from build123d import *

# Parameters (mm, degrees)
BOSS_EXTRUDE1_DEPTH       = 280
SKETCH4_R                 = 15
BOSS_EXTRUDE2_DEPTH       = 15
CUT_EXTRUDE1_DEPTH        = 15
CUT_EXTRUDE2_DEPTH        = 15
SKETCH9_R                 = 15
CUT_EXTRUDE3_DEPTH        = 15
LPATTERN1_COUNT           = 2
LPATTERN1_PITCH           = 180
LPATTERN2_COUNT           = 2
LPATTERN2_PITCH           = 220
LPATTERN2_COPY_1_SKETCH_R = 15
LPATTERN2_COPY_1_DEPTH    = 15


with BuildPart() as part:
    # Sketch1 → Boss-Extrude1 (new body)
    with BuildSketch(Plane.XY):
        with BuildLine():
            Line((-120, 0), (120, 0))
            Line((120, 0), (120, 15))
            Line((120, 15), (37.749172176, 15))
            ThreePointArc((37.749172176, 15), (54.444104817, 62.799964787), (25, 103.989794856))
            Line((25, 103.989794856), (10, 103.989794856))
            Line((10, 103.989794856), (10, 93.729833462))
            ThreePointArc((10, 93.729833462), (0, 15), (-10, 93.729833462))
            Line((-10, 93.729833462), (-10, 103.989794856))
            Line((-10, 103.989794856), (-25, 103.989794856))
            ThreePointArc((-25, 103.989794856), (-54.444104817, 62.799964787), (-37.749172176, 15))
            Line((-37.749172176, 15), (-120, 15))
            Line((-120, 15), (-120, 0))
        make_face()
    extrude(amount=BOSS_EXTRUDE1_DEPTH)

    # Sketch4 → Boss-Extrude2 (add)
    with BuildSketch(Plane(origin=(-10, 0, 0), x_dir=(0, 0, -1), z_dir=(1, 0, 0))):
        with BuildLine():
            Line((-258.604852185, 154.832655732), (-258.604852185, 103.989794856))
            Line((-258.604852185, 103.989794856), (-198.604852185, 103.989794856))
            Line((-198.604852185, 103.989794856), (-198.604852185, 154.832655732))
            ThreePointArc((-198.604852185, 154.832655732), (-228.604852185, 184.832655732), (-258.604852185, 154.832655732))
        make_face()
        with Locations((-228.604852185, 154.832655732)):
            Circle(SKETCH4_R, mode=Mode.SUBTRACT)
        with BuildLine():
            Line((-81.395147815, 103.989794856), (-21.395147815, 103.989794856))
            Line((-21.395147815, 103.989794856), (-21.395147815, 154.832655732))
            ThreePointArc((-21.395147815, 154.832655732), (-51.395147815, 184.832655732), (-81.395147815, 154.832655732))
            Line((-81.395147815, 154.832655732), (-81.395147815, 103.989794856))
        make_face()
        with Locations((-51.395147815, 154.832655732)):
            Circle(SKETCH4_R, mode=Mode.SUBTRACT)
    boss_extrude2 = extrude(amount=-BOSS_EXTRUDE2_DEPTH)

    # Mirror1: Boss-Extrude2 across plane
    add(boss_extrude2.mirror(Plane(origin=(0, 0, 0), x_dir=(0, 0, 1), z_dir=(1, 0, 0))))

    # Sketch5 → Cut-Extrude1 (cut)
    with BuildSketch(Plane(origin=(0, 15, 0), x_dir=(1, 0, 0), z_dir=(0, 1, 0))):
        with BuildLine():
            Line((120, -250), (120, -30.000000185))
            ThreePointArc((120, -30.000000185), (111.21320337, -51.213203501), (90, -60))
            Line((90, -60), (37.749172176, -60))
            Line((37.749172176, -60), (37.749172176, -220))
            Line((37.749172176, -220), (90, -220))
            ThreePointArc((90, -220), (111.213203436, -228.786796564), (120, -250))
        make_face()
        with BuildLine():
            Line((120, 0), (90, 0))
            ThreePointArc((90, 0), (111.213203501, -8.78679663), (120, -30.000000185))
            Line((120, -30.000000185), (120, 0))
        make_face()
        with BuildLine():
            Line((120, -280), (120, -250))
            ThreePointArc((120, -250), (111.213203436, -271.213203436), (90, -280))
            Line((90, -280), (120, -280))
        make_face()
    extrude(amount=-CUT_EXTRUDE1_DEPTH, mode=Mode.SUBTRACT)

    # Sketch7 → Cut-Extrude2 (cut)
    with BuildSketch(Plane(origin=(0, 15, 0), x_dir=(1, 0, 0), z_dir=(0, 1, 0))):
        with BuildLine():
            Line((-37.749172176, -220), (-37.749172176, -60))
            Line((-37.749172176, -60), (-90, -60))
            ThreePointArc((-90, -60), (-111.213203468, -51.213203403), (-120, -29.999999908))
            Line((-120, -29.999999908), (-120, -250))
            ThreePointArc((-120, -250), (-111.213203436, -228.786796564), (-90, -220))
            Line((-90, -220), (-37.749172176, -220))
        make_face()
        with BuildLine():
            ThreePointArc((-120, -29.999999908), (-111.213203403, -8.786796532), (-90, 0))
            Line((-90, 0), (-120, 0))
            Line((-120, 0), (-120, -29.999999908))
        make_face()
        with BuildLine():
            ThreePointArc((-90, -280), (-111.213203436, -271.213203436), (-120, -250))
            Line((-120, -250), (-120, -280))
            Line((-120, -280), (-90, -280))
        make_face()
    extrude(amount=-CUT_EXTRUDE2_DEPTH, mode=Mode.SUBTRACT)

    # Sketch9 → Cut-Extrude3 (cut)
    with BuildSketch(Plane(origin=(0, 15, 0), x_dir=(1, 0, 0), z_dir=(0, 1, 0))):
        with Locations((90, -30)):
            Circle(SKETCH9_R)
    cut_extrude3 = extrude(amount=-CUT_EXTRUDE3_DEPTH, mode=Mode.SUBTRACT)

    # LPattern1: Cut-Extrude3 ×2
    with Locations(*[(-i * LPATTERN1_PITCH, 0, 0) for i in range(1, LPATTERN1_COUNT)]):
        add(cut_extrude3, mode=Mode.SUBTRACT)

    # LPattern2: Cut-Extrude3 ×2
    with Locations(*[(0, 0, i * LPATTERN2_PITCH) for i in range(1, LPATTERN2_COUNT)]):
        add(cut_extrude3, mode=Mode.SUBTRACT)

    # LPattern2 copy 1 sketch → LPattern2 copy 1 (cut)
    with BuildSketch(Plane(origin=(-180, 15, 220), x_dir=(1, 0, 0), z_dir=(0, 1, 0))):
        with Locations((90, -30)):
            Circle(LPATTERN2_COPY_1_SKETCH_R)
    extrude(amount=-LPATTERN2_COPY_1_DEPTH, mode=Mode.SUBTRACT)


solid = part.part
Geometry: final body of the model. Coordinates: model frame, mm. A direction names the side the tool comes from. Round coordinates to 2 decimals unless told otherwise and drop trailing zeros. Loops run counter-clockwise (first coordinate to the right, second up) from the corner with the lowest first, then second, coordinate; pieces in that order, holes last. Notation, with made-up numbers: M 70.25,67 L 93.25,67 A24 ccw 93.25,98 Z; hole C -21.75,-34 d6. An arc over 180 degrees is marked long. One line per question, with ' | ' between items.
(1) Cut plane A-A on y = 55. Return the cut outline in (x, z).
Check result:
outline: M -55,0 L -40,0 L -40,280 L -55,280 Z; M 40,0 L 55,0 L 55,280 L 40,280 Z
(2) Cut plane D-D on y = 146.5. Give the number of separate pieces and of enclosed holes in the cut face, plus the area to 3 significant figures.
Check result:
separate pieces: 8 | enclosed holes: 0 | area: 2,100 mm2
(3) Cut plane B-B on z = 106. Return the cut outline in (x, y), plus the area to 3 significant figures.
Check result:
outline: M -37.75,0 L 37.75,0 L 37.75,15 A55 ccw 25,103.99 L 10,103.99 L 10,93.73 A40 cw long -10,93.73 L -10,103.99 L -25,103.99 A55 ccw -37.75,15 Z | area: 4,440 mm2
(4) Cut plane C-C on x = 82. Return the cut outline in (y, z).
Check result:
outline: M 0,0 L 15,0 L 15,17.31 L 0,17.31 Z; M 0,42.69 L 15,42.69 L 15,60 L 0,60 Z; M 0,220 L 15,220 L 15,237.31 L 0,237.31 Z; M 0,262.69 L 15,262.69 L 15,280 L 0,280 Z
(5) Access query for faces 1 (the flat face through (-25, 136, 229)), 2 (the flat face through (18, 103.99, 139)), 3 (the flat face through (-69, 15, 250)), 4 (the flat face through (-17, 130, 258.605)). Directions: +Z, -Z, +X, -X, +Y, -Y. A direction counts if a zero-diameter tool reaches every point of the face in a straight line with its end or side. Return the directions, or none.
Check result:
face 1: +Z, -Z, -X, +Y | face 2: +X, -X, +Y | face 3: +Z, -Z, -X | face 4: +Z, +X, -X, +Y
(6) Pull-direction query (X, two-part tool) for faces 5 (the flat face through (10, 99, 138)), 6 (the flat face through (37.749, 8, 139)), 7 (the flat face through (-37.749, 8, 141)); classes: +X half, -X half, draft (parallel to the pull), parting line (faces both ways), or undercut.
Check result:
face 5: undercut | face 6: +X half | face 7: -X half
(7) Material intervals for line 1 along Z through (x, y) = (-90, 9); line 2 along Z through (x, y) = (-15, 123); line 3 along Y through (x, z) = (24, 63.5), sorted ascending. Write a range as from..to.
Check result:
line 1: z = 0..15, 45..60, 220..235, 265..280 | line 2: z = 21.4..81.4, 198.6..258.6 | line 3: y = 0..23, 87..145.97, 163.69..182.28
(8) Contact query for flat-ended pins moving along their axis: P1, Ø4.5, axis at y = 9, z = 149, coming from the -X side; P2, Ø5, axis at x = 17, z = 89, coming from the +Y side; P3, Ø7.5, axis at x = 17, y = 121, coming from the -Z side. Output: stop coordinate, or through.
Check result:
P1: stops at x = -37.75 | P2: stops at y = 103.99 | P3: stops at z = 21.4
